Autodesk Inventor part; units mm, degrees
ref_plane "YZ Plane" through (0, 0, 0) normal (1, 0, 0) x (0, 1, 0)
ref_plane "XZ Plane" through (0, 0, 0) normal (0, 1, 0) x (-1, 0, 0)
ref_plane "XY Plane" through (0, 0, 0) normal (0, 0, 1) x (1, 0, 0)
sketch "Sketch1" plane through (0, 0, 0) normal (0, 0, 1) x (1, 0, 0)
  line L0 (0, 1490) -> (-122.2022, 1490)
  line L1 (-122.2022, 1490) -> (-122.2022, 0)
  line L2 (-122.2022, 0) -> (0, 0)
  line L3 (0, 0) -> (0, 1490)
  line L4 (-122.2022, 100) -> (-66, 100)
  line L5 (-66, 100) -> (-66, 105)
  line L6 (-66, 105) -> (-122.2022, 105)
  line L7 (-122.2022, 105) -> (-122.2022, 100)
  line L8 (-122.2022, 596.6667) -> (-66, 596.6667)
  line L9 (-66, 596.6667) -> (-66, 601.6667)
  line L10 (-66, 601.6667) -> (-122.2022, 601.6667)
  line L11 (-122.2022, 601.6667) -> (-122.2022, 596.6667)
  line L12 (-122.2022, 1093.3333) -> (-66, 1093.3333)
  line L13 (-66, 1093.3333) -> (-66, 1098.3333)
  line L14 (-66, 1098.3333) -> (-122.2022, 1098.3333)
  line L15 (-122.2022, 1098.3333) -> (-122.2022, 1093.3333)
  circle A0 centre (-122.2022, 1335) radius 30
  point P0 (-122.2022, 1098.3333)
  point P1 (-122.2022, 1093.3333)
  point P2 (-122.2022, 601.6667)
  point P3 (-122.2022, 596.6667)
  point P4 (-122.2022, 105)
  point P5 (-122.2022, 1365)
  point P6 (-122.2022, 1305)
  dimension "d0" = 1490
  dimension "d1" = 122.2022
  dimension "d2" = 5
  dimension "d4" = 100
  dimension "d7" = 496.6667
  dimension "d23" = 66
  dimension "d29" = 60
  dimension "d30" = 1335
extrude "Plate1" add sketch "Sketch1" along normal blind 4 contours L3 L2 L1 L4 L5 L6 L8 L9 L10 L12 L13 L14 A0 L0
chamfer "Corner Chamfer1" distance 3 angle 45 6 edges at (-122.2022, 100, 2) (-122.2022, 105, 2) (-122.2022, 596.6667, 2) (-122.2022, 601.6667, 2) (-122.2022, 1098.3333, 2) (-122.2022, 1093.3333, 2)
equation "\"d0\" = Стрингер_длина"
equation "\"d1\" = стрингер_глубина_7"
equation "\"d2\" = паз_под_стрингер_толщина"
equation "\"d7\" = Шаг_шпангоутов"
equation "\"d23\" = паз_под_стрингер_глубина - Thickness"
equation "\"d29\" = 2 * радиус_выреза_под_сварку"
equation "\"d12\" = Thickness"
equation "\"BendRadius\" = Thickness"
equation "\"BendReliefWidth\" = Thickness"
equation "\"BendReliefDepth\" = 0.5 * Thickness"
equation "\"CornerReliefSize\" = 4 * Thickness"
equation "\"MinimumRemnant\" = 2 * Thickness"
equation "\"TransitionRadius\" = BendRadius"
equation "\"JacobiRadiusSize\" = BendRadius"
equation "\"GapSize\" = Thickness"
properties part number "01013 GBK stringer C7" material "Steel"
Geometry check sheet. Reference: the model listing, model coordinates, mm. Round coordinates to 2 decimals unless told otherwise and drop trailing zeros. Write each loop counter-clockwise with the first axis right and the second up, starting at its lowest first coordinate (ties: lowest second). Pieces come first, ordered by that corner, then holes. Notation, with made-up numbers: (-38, 78.5) - (-19, 78.5) arc R25 cw to (-19, 114.5) - close; hole circle Ø10 at (49.25, -27.75). An arc over 180 degrees is marked (long way). One line per item, written item: value.
1. Scan lines: L1, parallel to Y at x = -72.5, z = 2; L2, parallel to Y at x = -108, z = 2.15; L3, parallel to Y at x = -98.5, z = 1.75. Record each from-to range of solid material in increasing order.
The answers:
L1: y = 0 to 100, 105 to 596.67, 601.67 to 1093.33, 1098.33 to 1490
L2: y = 0 to 100, 105 to 596.67, 601.67 to 1093.33, 1098.33 to 1308.57, 1361.43 to 1490
L3: y = 0 to 100, 105 to 596.67, 601.67 to 1093.33, 1098.33 to 1316.61, 1353.39 to 1490
2. Depth check by flat-ended pin: pin 1 Ø2 at (y, z) = (1095, 3) entering from -X. Enter the tip coordinate at first touch or a pass-through.
The answers:
pin 1: stops at x = -66
3. Cross-section at A-A on y = 1335. Record the boundary of the cut face in (x, z).
The answers:
outline: (-92.2, 0) - (0, 0) - (0, 4) - (-92.2, 4) - close
4. Mould release check, pull along Y, two halves, no side actions. Record for faces 1 (the face through (-92.21, 1335.66, 1.97)), 2 (the face through (-62, 755, 0)): released by +Y, released by -Y, zero draft, split by the parting line, or undercut.
The answers:
face 1: undercut
face 2: zero draft
